Geometry check sheet. Reference: the model listing, model coordinates, mm. Face numbers are marked on the shaded views. Give positions to 0.01 mm unless a question says otherwise; leave off trailing zeros. Loops run counter-clockwise (first coordinate to the right, second up) from the corner with the lowest first, then second, coordinate; pieces in that order, holes last. Notation, with made-up numbers: (88, -20) -> (95, -20) arc R18 ccw to (95, 9) -> close; hole circle Ø5 at (-26.5, 9.25). An arc over 180 degrees is marked (long way). One line per question, with ' | ' between items.
Autodesk Inventor part; units mm, degrees
ref_plane "YZ Plane" through (0, 0, 0) normal (1, 0, 0) x (0, 1, 0)
ref_plane "XZ Plane" through (0, 0, 0) normal (0, 1, 0) x (-1, 0, 0)
ref_plane "XY Plane" through (0, 0, 0) normal (0, 0, 1) x (1, 0, 0)
sketch "Sketch1" plane through (0, 0, 0) normal (0, 0, 1) x (1, 0, 0)
  circle A0 centre (-2.413, 0) radius 2.413
  line L0 (-1.2065, -2.0897) -> (-3.6195, -2.0897)
  line L1 (-3.6195, -2.0897) -> (-4.826, 0)
  line L2 (-4.826, 0) -> (-3.6195, 2.0897)
  line L3 (-3.6195, 2.0897) -> (-1.2065, 2.0897)
  line L4 (-1.2065, 2.0897) -> (0, 0)
  line L5 (0, 0) -> (-1.2065, -2.0897)
  circle A1 centre (-2.413, 0) radius 1.05
  line L6 (-1.913, -3.5) -> (-9.8027, -3.5)
  point P0 (0, 0)
  dimension "d0" = 2.1
extrude "Extrusion1" add sketch "Sketch1" against normal blind 10 contours L5 L0 L1 L2 L3 L4
properties part number "SpacerShiel"
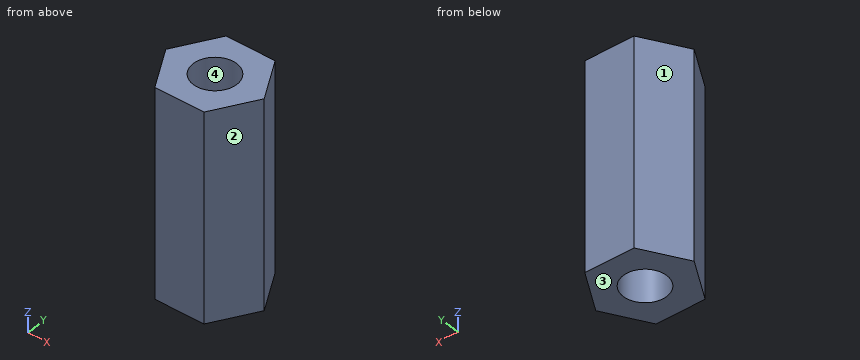
Item 1: Release check for a two-part mould opening along X. For the marked faces 1, 2, 3 and 4 record: pulls with the +X half, pulls with the -X half, needs draft (parallel to the pull), parting line crosses it, or undercut.
Result:
face 1: pulls with the -X half | face 2: pulls with the +X half | face 3: needs draft | face 4: undercut
Item 2: Sectioned sample at C-C (y = 0.5). Record the cut outline in (x, z), plus the area to 3 significant figures.
Result:
outline: (-4.54, -10) -> (-3.34, -10) -> (-3.34, 0) -> (-4.54, 0) -> close; (-1.49, -10) -> (-0.29, -10) -> (-0.29, 0) -> (-1.49, 0) -> close | area: 24.0 mm2
Item 3: Sectioned sample at B-B (x = -2.7). Record the cut outline in (y, z), plus the area to 3 significant figures.
Result:
outline: (-2.09, -10) -> (-1.01, -10) -> (-1.01, 0) -> (-2.09, 0) -> close; (1.01, -10) -> (2.09, -10) -> (2.09, 0) -> (1.01, 0) -> close | area: 21.6 mm2
Item 4: Sectioned sample at D-D (x = -1.05). Record the cut outline in (y, z).
Result:
outline: (-1.82, -10) -> (1.82, -10) -> (1.82, 0) -> (-1.82, 0) -> close
Item 5: Sectioned sample at A-A (z = -6). Record the cut outline in (x, y), plus the area to 3 significant figures.
Result:
outline: (-4.83, 0) -> (-3.62, -2.09) -> (-1.21, -2.09) -> (0, 0) -> (-1.21, 2.09) -> (-3.62, 2.09) -> close; hole circle Ø2.1 at (-2.41, 0) | area: 11.7 mm2
Item 6: Scan lines: probe 1 along Y at (x, z) = (-1.65, -5.25); probe 2 along Y at (x, z) = (-2.5, -7.25); probe 3 along X at (y, z) = (-0.9, -3). Record each from-to range of solid material in increasing order.
Result:
probe 1: -2.09 to -0.72, 0.72 to 2.09 | probe 2: -2.09 to -1.05, 1.05 to 2.09 | probe 3: -4.31 to -2.95, -1.87 to -0.52
